```python
from build123d import *

# Parameters (mm, degrees)
SKETCH1_R               = 35.75
OUTERCASE_DEPTH         = 25
SKETCH2_R               = 35
CUT_EXTRUDE1_DEPTH      = 15
SKETCH3_R               = 4.7625
BEARING_DEPTH           = 3.175
SKETCH4_R               = 3.429
SHAFT_ROOM_DEPTH        = 5
CUT_EXTRUDE4_DEPTH      = 56.616594871
CUT_EXTRUDE4_DEPTH_BACK = 56.616594871
FILLET1_R               = 0.7
FILLET2_R               = 1.2


with BuildPart() as part:
    # Sketch1 → OuterCase (new body)
    with BuildSketch(Plane.XY):
        Circle(SKETCH1_R)
    extrude(amount=OUTERCASE_DEPTH)

    # Sketch2 → Cut-Extrude1 (cut)
    with BuildSketch(Plane.XY.offset(25)):
        Circle(SKETCH2_R)
    extrude(amount=-CUT_EXTRUDE1_DEPTH, mode=Mode.SUBTRACT)

    # Sketch3 → Bearing (cut)
    with BuildSketch(Plane.XY.offset(10)):
        Circle(SKETCH3_R)
    extrude(amount=-BEARING_DEPTH, mode=Mode.SUBTRACT)

    # Sketch4 → Shaft_Room (cut)
    with BuildSketch(Plane.XY.offset(6.825)):
        Circle(SKETCH4_R)
    extrude(amount=-SHAFT_ROOM_DEPTH, mode=Mode.SUBTRACT)

    # Sketch6 → Cut-Extrude4 (cut, two sides: drawn at the far end of the back side and taken through both)
    with BuildSketch(Plane.XY.offset(1.825).offset(-CUT_EXTRUDE4_DEPTH_BACK)):
        with BuildLine():
            ThreePointArc((19.303315658, -22.734538204), (22.163629102, -19.95622128), (24.627741947, -16.821163733))
            Line((24.627741947, -16.821163733), (8.05540901, -7.253122851))
            Line((8.05540901, -7.253122851), (19.303315658, -22.734538204))
        make_face()
        with BuildLine():
            ThreePointArc((26.881426088, -12.917668297), (28.364409143, -9.216155203), (29.340345457, -5.349892635))
            Line((29.340345457, -5.349892635), (10.30909315, -3.349627415))
            Line((10.30909315, -3.349627415), (26.881426088, -12.917668297))
        make_face()
        with BuildLine():
            ThreePointArc((8.387486585, -28.620399919), (12.130556239, -27.245675401), (15.656778118, -25.383902807))
            Line((15.656778118, -25.383902807), (4.40887147, -9.902487453))
            Line((4.40887147, -9.902487453), (8.387486585, -28.620399919))
        make_face()
        with BuildLine():
            ThreePointArc((-3.978615115, -29.55753448), (0, -29.824104727), (3.978615115, -29.55753448))
            Line((3.978615115, -29.55753448), (0, -10.839622014))
            Line((0, -10.839622014), (-3.978615115, -29.55753448))
        make_face()
        with BuildLine():
            ThreePointArc((-15.656778118, -25.383902807), (-12.130556239, -27.245675401), (-8.387486585, -28.620399919))
            Line((-8.387486585, -28.620399919), (-4.40887147, -9.902487453))
            Line((-4.40887147, -9.902487453), (-15.656778118, -25.383902807))
        make_face()
        with BuildLine():
            ThreePointArc((-24.627741947, -16.821163733), (-22.163629102, -19.95622128), (-19.303315658, -22.734538204))
            Line((-19.303315658, -22.734538204), (-8.05540901, -7.253122851))
            Line((-8.05540901, -7.253122851), (-24.627741947, -16.821163733))
        make_face()
        with BuildLine():
            ThreePointArc((-29.340345457, -5.349892635), (-28.364409143, -9.216155203), (-26.881426088, -12.917668297))
            Line((-26.881426088, -12.917668297), (-10.30909315, -3.349627415))
            Line((-10.30909315, -3.349627415), (-29.340345457, -5.349892635))
        make_face()
        with BuildLine():
            ThreePointArc((-28.979736689, 7.046423503), (-29.66072516, 3.117467835), (-29.811493737, -0.867216188))
            Line((-29.811493737, -0.867216188), (-10.78024143, 1.133049031))
            Line((-10.78024143, 1.133049031), (-28.979736689, 7.046423503))
        make_face()
        with BuildLine():
            ThreePointArc((-23.608268175, 18.224349002), (-25.828432338, 14.912052363), (-27.58688329, 11.333185478))
            Line((-27.58688329, 11.333185478), (-9.387388031, 5.419811007))
            Line((-9.387388031, 5.419811007), (-23.608268175, 18.224349002))
        make_face()
        with BuildLine():
            ThreePointArc((-14.154715619, 26.251118995), (-17.530168921, 24.128207566), (-20.592250104, 21.573976416))
            Line((-20.592250104, 21.573976416), (-6.37136996, 8.769438422))
            Line((-6.37136996, 8.769438422), (-14.154715619, 26.251118995))
        make_face()
        with BuildLine():
            Line((-2.253684141, 10.602750266), (-2.253684141, 29.738832031))
            ThreePointArc((-2.253684141, 29.738832031), (-6.200780041, 29.172376482), (-10.037029799, 28.084430839))
            Line((-10.037029799, 28.084430839), (-2.253684141, 10.602750266))
        make_face()
        with BuildLine():
            ThreePointArc((10.037029799, 28.084430839), (6.200780041, 29.172376482), (2.253684141, 29.738832031))
            Line((2.253684141, 29.738832031), (2.253684141, 10.602750266))
            Line((2.253684141, 10.602750266), (10.037029799, 28.084430839))
        make_face()
        with BuildLine():
            ThreePointArc((20.592250104, 21.573976416), (17.530168921, 24.128207566), (14.154715619, 26.251118995))
            Line((14.154715619, 26.251118995), (6.37136996, 8.769438422))
            Line((6.37136996, 8.769438422), (20.592250104, 21.573976416))
        make_face()
        with BuildLine():
            ThreePointArc((27.58688329, 11.333185478), (25.828432338, 14.912052363), (23.608268175, 18.224349002))
            Line((23.608268175, 18.224349002), (9.387388031, 5.419811007))
            Line((9.387388031, 5.419811007), (27.58688329, 11.333185478))
        make_face()
        with BuildLine():
            ThreePointArc((29.811493737, -0.867216188), (29.66072516, 3.117467835), (28.979736689, 7.046423503))
            Line((28.979736689, 7.046423503), (10.78024143, 1.133049031))
            Line((10.78024143, 1.133049031), (29.811493737, -0.867216188))
        make_face()
    extrude(amount=CUT_EXTRUDE4_DEPTH + CUT_EXTRUDE4_DEPTH_BACK, mode=Mode.SUBTRACT)

    # Fillet1
    fillet1_edges = [part.edges().sort_by_distance(p)[0] for p in [
        (-4.40887147, -9.902487453, 5),
        (0, -10.839622014, 5),
        (10.30909315, -3.349627415, 5),
        (4.40887147, -9.902487453, 5),
        (9.387388031, 5.419811007, 5),
        (10.78024143, 1.133049031, 5),
        (2.253684141, 10.602750266, 5),
        (6.37136996, 8.769438422, 5),
        (-6.37136996, 8.769438422, 5),
        (-2.253684141, 10.602750266, 5),
        (8.05540901, -7.253122851, 5),
        (-10.78024143, 1.133049031, 5),
        (-9.387388031, 5.419811007, 5),
        (-8.05540901, -7.253122851, 5),
        (-10.30909315, -3.349627415, 5),
    ]]
    fillet(fillet1_edges, radius=FILLET1_R)

    # Fillet2
    fillet2_edges = [part.edges().sort_by_distance(p)[0] for p in [
        (-26.881426088, -12.917668297, 5),
        (-15.656778118, -25.383902807, 5),
        (-8.387486585, -28.620399919, 5),
        (-3.978615115, -29.55753448, 5),
        (3.978615115, -29.55753448, 5),
        (26.881426088, -12.917668297, 5),
        (29.340345457, -5.349892635, 5),
        (8.387486585, -28.620399919, 5),
        (15.656778118, -25.383902807, 5),
        (27.58688329, 11.333185478, 5),
        (23.608268175, 18.224349002, 5),
        (29.811493737, -0.867216188, 5),
        (28.979736689, 7.046423503, 5),
        (10.037029799, 28.084430839, 5),
        (2.253684141, 29.738832031, 5),
        (20.592250104, 21.573976416, 5),
        (14.154715619, 26.251118995, 5),
        (-14.154715619, 26.251118995, 5),
        (-20.592250104, 21.573976416, 5),
        (-2.253684141, 29.738832031, 5),
        (-10.037029799, 28.084430839, 5),
        (19.303315658, -22.734538204, 5),
        (24.627741947, -16.821163733, 5),
        (-28.979736689, 7.046423503, 5),
        (-29.811493737, -0.867216188, 5),
        (-23.608268175, 18.224349002, 5),
        (-27.58688329, 11.333185478, 5),
        (-24.627741947, -16.821163733, 5),
        (-19.303315658, -22.734538204, 5),
        (-29.340345457, -5.349892635, 5),
    ]]
    fillet(fillet2_edges, radius=FILLET2_R)


solid = part.part
```
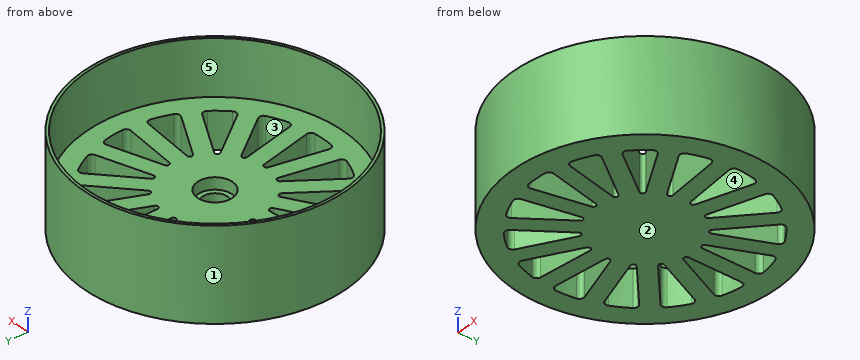
Input: part model. Units: mm. Frame: model coordinates. Face numbers are marked on the shaded views. A direction names the side the tool comes from. Give positions to 0.01 mm unless a question says otherwise; leave off trailing zeros. Order: outer loops, then holes, each group sorted by start corner. A loop starts at its lowest first (then second) coordinate and runs counter-clockwise, first axis right, second up.
1. Reachability of the marked faces 4 and 5 from +Z, -Z, +X, -X, +Y, -Y: full face, straight path, thin tool, end or side. Return the list, or none.
Derived:
face 4: +Z, -Z
face 5: +Z
2. Pin query (flat end, axial travel): pin 1 (10 mm diameter, centred on x = 8.5, z = 16.5, fed in from +Y); pin 2 (2 mm diameter, centred on x = -1, y = 1, fed in from +Z) (3 decimals); pin 3 (5 mm diameter, centred on y = 27, z = 15, fed in from -X). Return the tip coordinate at first contact, or that it passes through.
Derived:
pin 1: stops at y = 35.58
pin 2: stops at z = 1.825
pin 3: stops at x = -26.03
3. Material intervals for L1, parallel to Y at x = 0, z = 7.95; L2, parallel to X at y = -11, z = 3.25; L3, parallel to X at y = -27.5, z = 6.25, sorted ascending.
Derived:
L1: y = -35.75 to -29.82, -13.51 to -4.76, 4.76 to 35.75
L2: x = -34.02 to -27.72, -23.56 to -14.55, -10.78 to 10.78, 14.55 to 23.56, 27.72 to 34.02
L3: x = -22.84 to -11.54, -8.16 to -3.54, 3.54 to 8.16, 11.54 to 22.84
4. Mould query, pull axis Y, two halves, no side actions, for the marked faces 1, 2 and 3. Classes: released by +Y, released by -Y, zero draft, split by the parting line, or undercut.
Derived:
face 1: split by the parting line
face 2: zero draft
face 3: undercut
5. Section A-A on x = 31. Return the cut outline in (y, z), and give its area (3 significant figures).
Derived:
outline: (-17.81, 0) - (17.81, 0) - (17.81, 25) - (16.25, 25) - (16.25, 10) - (-16.25, 10) - (-16.25, 25) - (-17.81, 25) - close
area: 403 mm2
